Here's how the part is built. I have some questions about the finished solid (model axes, mm). A direction names the side the tool comes from. Round coordinates to 2 decimals unless told otherwise and drop trailing zeros. Write each loop counter-clockwise with the first axis right and the second up, starting at its lowest first coordinate (ties: lowest second). Pieces come first, ordered by that corner, then holes. Notation, with made-up numbers: (3.5, -6.5) -> (21.5, -6.5) arc R28 ccw to (21.5, 25.5) -> close; hole circle Ø5 at (89, 58.25). An arc over 180 degrees is marked (long way). Put each result on its own line as item: value. Start each with the question number.
1) I want a section at B-B, the plane z = -82. List the corners of the cut face in (x, y) for me.
2) I want a section at D-D, the plane z = -1. List the corners of the cut face in (x, y) for me.
3) I want a section at A-A, the plane y = 64. List the corners of the cut face in (x, z) for me.
4) We'd pull the mould along Z, two halves only. Please class faces 6 (the flat face through (-5, 1, 220)), 7 (the flat face through (0, -74.372, 196)), 8 (the flat face through (41, -4.05, -87)), 9 (the flat face through (0, -8, -325)): released by +Z, released by -Z, zero draft, split by the parting line, or undercut.
5) I want a section at C-C, the plane x = -19. List the corners of the cut face in (y, z) for me.
6) Which directions (+Z, -Z, +X, -X, +Y, -Y) give clear straight access to the entire face, cutting with the end or side of a thin tool? Please do faces 1 (the flat face through (99.848, -86, 69)), 2 (the flat face through (-97.181, -85, 66)), 3 (the flat face through (-86, -92.092, -81)), 4 (the cylindrical face through (7.836, 0.345, -255.487)), 5 (the flat face through (-41, 4.05, -87)).
7) If I drill on line 1 along X through (y, z) = (71.5, -119); line 2 along Z through (x, y) = (-2, 46.5); line 3 along Y through (x, z) = (0, -240), over which ranges is the centre line in solid material (lowest first)? Write a range as [from, to].
8) Will these pins go through, and if not, where does the flat tip stop? P1, Ø6, axis at x = -75.5, y = -70, coming from the +Z side; P2, Ø8, axis at x = 36, z = -50, coming from the -Y side; P3, Ø10, axis at x = -27, y = -48, coming from the -Z side; P4, Ø15, axis at x = -8.5, y = 87.5, coming from the +Z side.
from build123d import *

# Parameters (mm, degrees)
BOSS_EXTRUDE1_DEPTH      = 175
BOSS_EXTRUDE1_DEPTH_BACK = 325
SKETCH1_R                = 12.637842641
BOSS_EXTRUDE2_DEPTH      = 100
BOSS_EXTRUDE2_DEPTH_BACK = 100
SKETCH2_W                = 5.637667912
SKETCH2_H                = 67.983642473
BOSS_EXTRUDE3_DEPTH      = 100
BOSS_EXTRUDE3_DEPTH_BACK = 100
SKETCH3_W                = 67.983642473
SKETCH3_H                = 29.694964858
SKETCH4_W                = 193.517193279
SKETCH4_H                = 18.701241368
CUT_EXTRUDE1_DEPTH       = 63
BOSS_EXTRUDE4_DEPTH      = 100
BOSS_EXTRUDE4_DEPTH_BACK = 100
SKETCH5_W                = 98.759478103
SKETCH5_H                = 8.09947515
BOSS_EXTRUDE5_DEPTH      = 100
BOSS_EXTRUDE5_DEPTH_BACK = 100
SKETCH6_W                = 30
SKETCH6_H                = 98.759478103
SKETCH7_W                = 22.635129566
SKETCH7_H                = 191.944809052
CUT_EXTRUDE2_DEPTH       = 86
SKETCH8_W                = 150
SKETCH8_H                = 150
BOSS_EXTRUDE6_DEPTH      = 5
BOSS_EXTRUDE7_REACH      = 566.29
SKETCH10_W               = 21.396607864
SKETCH10_H               = 165.105210234
SKETCH11_W               = 33.062075252
SKETCH11_H               = 149.372216897
CUT_EXTRUDE3_DEPTH       = 40
SKETCH12_W               = 8
SKETCH12_H               = 30
CUT_EXTRUDE4_DEPTH       = 30
SKETCH13_R               = 7.843556452
CUT_EXTRUDE5_DEPTH       = 141
SKETCH14_W               = 29
SKETCH14_H               = 9
CUT_EXTRUDE6_DEPTH       = 141
SKETCH15_W               = 29
SKETCH15_H               = 9
CUT_EXTRUDE7_DEPTH       = 83


with BuildPart() as part:
    # Sketch1 → Boss-Extrude1 (new, two sides: drawn at the far end of the back side and taken through both)
    with BuildSketch(Plane.XY.offset(-BOSS_EXTRUDE1_DEPTH_BACK)):
        Circle(SKETCH1_R)
    extrude(amount=BOSS_EXTRUDE1_DEPTH + BOSS_EXTRUDE1_DEPTH_BACK)

    # Sketch2 → Boss-Extrude2 (add, two sides: drawn at the far end of the back side and taken through both)
    with BuildSketch(Plane(origin=(0, 0, 0), x_dir=(1, 0, 0), z_dir=(0, 1, 0)).offset(-BOSS_EXTRUDE2_DEPTH_BACK)):
        with Locations((0, -65.65046148)):
            Rectangle(SKETCH2_W, SKETCH2_H)
    extrude(amount=BOSS_EXTRUDE2_DEPTH + BOSS_EXTRUDE2_DEPTH_BACK)

    # Sketch3 → Boss-Extrude3 (add, two sides: drawn at the far end of the back side and taken through both)
    with BuildSketch(Plane(origin=(2.818833956, 0, 0), x_dir=(0, 0, -1), z_dir=(1, 0, 0)).offset(-BOSS_EXTRUDE3_DEPTH_BACK)):
        with Locations((-65.65046148, 85.152517571)):
            Rectangle(SKETCH3_W, SKETCH3_H)
        with Locations((-65.65046148, -85.152517571)):
            Rectangle(SKETCH3_W, SKETCH3_H)
    extrude(amount=BOSS_EXTRUDE3_DEPTH + BOSS_EXTRUDE3_DEPTH_BACK)

    # Sketch4 → Cut-Extrude1 (cut)
    with BuildSketch(Plane.XY.offset(99.642282717)):
        with Locations((3.08986644, 85.773498781)):
            Rectangle(SKETCH4_W, SKETCH4_H)
        with Locations((3.08986644, -85.773498781)):
            Rectangle(SKETCH4_W, SKETCH4_H)
    extrude(amount=-CUT_EXTRUDE1_DEPTH, mode=Mode.SUBTRACT)

    # Sketch5 → Boss-Extrude4 (add, two sides: drawn at the far end of the back side and taken through both)
    with BuildSketch(Plane(origin=(0, 0, 0), x_dir=(0, 0, -1), z_dir=(1, 0, 0)).offset(-BOSS_EXTRUDE4_DEPTH_BACK)):
        with Locations((88.14712325, 0)):
            Rectangle(SKETCH5_W, SKETCH5_H)
    extrude(amount=BOSS_EXTRUDE4_DEPTH + BOSS_EXTRUDE4_DEPTH_BACK)

    # Sketch6 → Boss-Extrude5 (add, two sides: drawn at the far end of the back side and taken through both)
    with BuildSketch(Plane(origin=(0, 4.049737575, 0), x_dir=(1, 0, 0), z_dir=(0, 1, 0)).offset(-BOSS_EXTRUDE5_DEPTH_BACK)):
        with Locations((-85, 88.14712325)):
            Rectangle(SKETCH6_W, SKETCH6_H)
        with Locations((85, 88.14712325)):
            Rectangle(SKETCH6_W, SKETCH6_H)
    extrude(amount=BOSS_EXTRUDE5_DEPTH + BOSS_EXTRUDE5_DEPTH_BACK)

    # Sketch7 → Cut-Extrude2 (cut)
    with BuildSketch(Plane.XY.offset(-38.767384198)):
        with Locations((-85.588690937, 3.879977002)):
            Rectangle(SKETCH7_W, SKETCH7_H)
        with Locations((85.588690937, 3.879977002)):
            Rectangle(SKETCH7_W, SKETCH7_H)
    extrude(amount=-CUT_EXTRUDE2_DEPTH, mode=Mode.SUBTRACT)

    # Sketch8 → Boss-Extrude6 (add)
    with BuildSketch(Plane.XY.offset(175)):
        Rectangle(SKETCH8_W, SKETCH8_H)
    extrude(amount=BOSS_EXTRUDE6_DEPTH)

    # Boss-Extrude7: up to this face of the body (flat: up to its plane)
    boss_extrude7_end = Plane(part.part.faces().sort_by_distance((0, -72.878679656, 175))[0])
    # Sketch10 → Boss-Extrude7 (add, up to the picked face)
    with BuildSketch(Plane.XY.offset(220), mode=Mode.PRIVATE) as boss_extrude7_sk1:
        Rectangle(SKETCH10_W, SKETCH10_H)
    boss_extrude7_tool1 = split(extrude(boss_extrude7_sk1.sketch, amount=-BOSS_EXTRUDE7_REACH, mode=Mode.PRIVATE), bisect_by=boss_extrude7_end, keep=Keep.BOTH, mode=Mode.PRIVATE)
    add(boss_extrude7_tool1.solids().sort_by(Axis((0, 0, 220), (0, 0, -1)))[0])

    # Sketch11 → Cut-Extrude3 (cut)
    with BuildSketch(Plane.ZY.offset(10.698303932)):
        with Locations((196.531037626, 0.313891551)):
            Rectangle(SKETCH11_W, SKETCH11_H)
    extrude(amount=-CUT_EXTRUDE3_DEPTH, mode=Mode.SUBTRACT)

    # Sketch12 → Cut-Extrude4 (cut)
    with BuildSketch(Plane.XY.offset(220)):
        Rectangle(SKETCH12_W, SKETCH12_H)
    extrude(amount=-CUT_EXTRUDE4_DEPTH, mode=Mode.SUBTRACT)

    # Sketch13 → Cut-Extrude5 (cut)
    with BuildSketch(Plane(origin=(0, 0, -325), x_dir=(-1, 0, 0), z_dir=(0, 0, -1))):
        Circle(SKETCH13_R)
    extrude(amount=-CUT_EXTRUDE5_DEPTH, mode=Mode.SUBTRACT)

    # Sketch14 → Cut-Extrude6 (cut)
    with BuildSketch(Plane.ZY):
        with Locations((-307.774546231, -0.108379214)):
            Rectangle(SKETCH14_W, SKETCH14_H)
    extrude(amount=-CUT_EXTRUDE6_DEPTH, mode=Mode.SUBTRACT)

    # Sketch15 → Cut-Extrude7 (cut)
    with BuildSketch(Plane.ZY):
        with Locations((-274.519862271, -0.063837762)):
            Rectangle(SKETCH15_W, SKETCH15_H)
    extrude(amount=CUT_EXTRUDE7_DEPTH, mode=Mode.SUBTRACT)


solid = part.part
Findings:
1. outline: (-100, -95.95) -> (-70, -95.95) -> (-70, -4.05) -> (-11.97, -4.05) arc R12.64 ccw to (11.97, -4.05) -> (70, -4.05) -> (70, -95.95) -> (100, -95.95) -> (100, 104.05) -> (70, 104.05) -> (70, 4.05) -> (11.97, 4.05) arc R12.64 ccw to (-11.97, 4.05) -> (-70, 4.05) -> (-70, 104.05) -> (-100, 104.05) -> close; hole (-96.91, -92.09) -> (-74.27, -92.09) -> (-74.27, 99.85) -> (-96.91, 99.85) -> close; hole (74.27, -92.09) -> (96.91, -92.09) -> (96.91, 99.85) -> (74.27, 99.85) -> close
2. outline: circle Ø25.28 at (0, 0)
3. outline: (-100, -137.53) -> (-70, -137.53) -> (-70, -38.77) -> (-74.27, -38.77) -> (-74.27, -124.77) -> (-96.91, -124.77) -> (-96.91, -38.77) -> (-100, -38.77) -> close; (-75, 175) -> (75, 175) -> (75, 180) -> (-75, 180) -> close; (-10.7, 213.06) -> (10.7, 213.06) -> (10.7, 220) -> (-10.7, 220) -> close; (-2.82, 31.66) -> (2.82, 31.66) -> (2.82, 99.64) -> (-2.82, 99.64) -> close; (70, -137.53) -> (100, -137.53) -> (100, -38.77) -> (96.91, -38.77) -> (96.91, -124.77) -> (74.27, -124.77) -> (74.27, -38.77) -> (70, -38.77) -> close
4. face 6: released by +Z
4. face 7: undercut
4. face 8: zero draft
4. face 9: released by -Z
5. outline: (-100, 31.66) -> (-70.31, 31.66) -> (-70.31, 99.64) -> (-76.42, 99.64) -> (-76.42, 36.64) -> (-95.12, 36.64) -> (-95.12, 99.64) -> (-100, 99.64) -> close; (-75, 175) -> (75, 175) -> (75, 180) -> (-75, 180) -> close; (-4.05, -137.53) -> (4.05, -137.53) -> (4.05, -38.77) -> (-4.05, -38.77) -> close; (70.31, 31.66) -> (100, 31.66) -> (100, 99.64) -> (95.12, 99.64) -> (95.12, 36.64) -> (76.42, 36.64) -> (76.42, 99.64) -> (70.31, 99.64) -> close
6. face 1: +Z
6. face 2: +Z, -X, +Y, -Y
6. face 3: none
6. face 4: -Z
6. face 5: -Z, +Y
7. line 1: x = [-100, -96.91], [-74.27, -70], [70, 74.27], [96.91, 100]
7. line 2: z = [31.66, 99.64], [175, 180], [213.06, 220]
7. line 3: y = [-12.64, -7.84], [7.84, 12.64]
8. P1: stops at z = 180
8. P2: stops at y = -4.05
8. P3: stops at z = 175
8. P4: stops at z = 220
